```python
from build123d import *

# Parameters (mm, degrees)
EXTRUSION1_DEPTH = 3


with BuildPart() as part:
    # Esquisse1 → Extrusion1 (new body)
    with BuildSketch(Plane(origin=(0, 0, 0), x_dir=(1, 0, 0), z_dir=(0, 1, 0))):
        with BuildLine():
            Line((80.5, 0), (-80.5, 0))
            Line((-80.5, 0), (-80.5, -83))
            Line((-80.5, -83), (-90.5, -83))
            Line((-90.5, -83), (-90.5, -96))
            Line((-90.5, -96), (-125.5, -96))
            Line((-125.5, -96), (-125.5, -196))
            Line((-125.5, -196), (-97.787187079, -212))
            ThreePointArc((-97.787187079, -212), (0, -161.553332366), (97.787187079, -212))
            Line((97.787187079, -212), (125.5, -196))
            Line((125.5, -196), (125.5, -96))
            Line((125.5, -96), (90.5, -96))
            Line((90.5, -96), (90.5, -83))
            Line((90.5, -83), (80.5, -83))
            Line((80.5, -83), (80.5, 0))
        make_face()
    extrude(amount=EXTRUSION1_DEPTH)


solid = part.part
```
Here's how the part is built. I have some questions about the finished solid (model axes, mm). Give positions to 0.01 mm unless a question says otherwise; leave off trailing zeros. Order: outer loops, then holes, each group sorted by start corner. A loop starts at its lowest first (then second) coordinate and runs counter-clockwise, first axis right, second up. Notation, with made-up numbers: (76.5, 41.5) - (107.5, 41.5) arc R12 cw to (107.5, 54.5) - close; hole circle Ø7 at (17.5, -38.5). An arc over 180 degrees is marked (long way). Answer as a JSON object with one key per item and string values. Group by question number.
Item 1: For P1, Ø1, axis at y = 2, z = 76.5, coming from the +X side; P2, Ø1.5, axis at y = 2, z = 88, coming from the -X side; P3, Ø0.9, axis at x = 115.5, y = 1, coming from the -Z side, each with a flat end and sliding along its axis, tell me the tip position at first contact or that it passes through.
Item 2: If we section it at D-D on x = 32: Please give me the cut outline in (y, z).
Item 3: If we section it at C-C on z = 14: Please give me the cut outline in (x, y), and give its area (3 significant figures).
Item 4: If we section it at B-B on z = 173: Please give me the cut outline in (x, y).
Item 5: Please list where these lines run through material, in increasing order: probe 1 along X at (y, z) = (2.6, 48); probe 2 along X at (y, z) = (2.95, 195); probe 3 along X at (y, z) = (0.4, 85.5).
Item 6: If we mould it in two halves opening along X, with no side actions, what happens to faces 1 (the flat face through (-111.838, 1.479, 203.888)), 2 (the flat face through (-2, 0, 105)), 3 (the flat face through (111.45, 1.48, 204.11)), 4 (the cylindrical face through (-1.6, 1.479, 161.564))? For each: pulls with the +X half, pulls with the -X half, needs draft (parallel to the pull), parting line crosses it, or undercut.
Item 7: If we section it at A-A on y = 1.15: Please give me the cut outline in (x, z), and give its area (3 significant figures).
Result set:
{
 "1": {"P1": "x = 80.5", "P2": "x = -90.5", "P3": "z = 96"},
 "2": {"outline": "(0, 0) - (3, 0) - (3, 165.9) - (0, 165.9) - close"},
 "3": {"outline": "(-80.5, 0) - (80.5, 0) - (80.5, 3) - (-80.5, 3) - close", "area": "483 mm²"},
 "4": {"outline": "(-125.5, 0) - (-51.15, 0) - (-51.15, 3) - (-125.5, 3) - close; (51.15, 0) - (125.5, 0) - (125.5, 3) - (51.15, 3) - close"},
 "5": {"probe 1": "-80.5 to 80.5", "probe 2": "-125.5 to -83.12, 83.12 to 125.5", "probe 3": "-90.5 to 90.5"},
 "6": {"face 1": "pulls with the -X half", "face 2": "needs draft", "face 3": "pulls with the +X half", "face 4": "undercut"},
 "7": {"outline": "(-125.5, 96) - (-90.5, 96) - (-90.5, 83) - (-80.5, 83) - (-80.5, 0) - (80.5, 0) - (80.5, 83) - (90.5, 83) - (90.5, 96) - (125.5, 96) - (125.5, 196) - (97.79, 212) arc R120 cw to (-97.79, 212) - (-125.5, 196) - close", "area": "37,500 mm²"}
}
